Source: CAD feature listing. Evaluate the final solid. Frame: model axes, mm. Face numbers are marked on the shaded views. A direction names the side the tool comes from. Give positions to 0.01 mm unless a question says otherwise; leave off trailing zeros. Order: outer loops, then holes, each group sorted by start corner. A loop starts at its lowest first (then second) coordinate and runs counter-clockwise, first axis right, second up.
1) Access query for the marked faces 4, 5 and 6. Directions: +Z, -Z, +X, -X, +Y, -Y. A direction counts if a zero-diameter tool reaches every point of the face in a straight line with its end or side. Return the directions, or none.
2) First-contact query: P1, Ø13.5, axis at x = 25.15, z = 123.69, coming from the +Y side; P2, Ø2, axis at x = -53.5, z = 72.5, coming from the +Y side; P3, Ø12, axis at y = 124, z = 5, coming from the -X side; P4, Ø8, axis at x = -12.5, y = 18, coming from the -Z side. Flat tips, straight axial feed; report the tip coordinate or a pass-through.
3) Material intervals for line 1 (Y direction, x = 25.5, z = 40); line 2 (Z direction, x = -10, y = 55.5); line 3 (X direction, y = 39.5, z = 27.5), sorted ascending.
4) Section B-B, the plane y = 42. Return loops of the section in (x, z).
5) Draft query along X for the marked faces 1, 2 and 3. Return one class per face: released by +X, released by -X, zero draft, split by the parting line, or undercut.
```python
from build123d import *

# Parameters (mm, degrees)
ESQUISSE1_W             = 170
ESQUISSE1_H             = 170
BOSS_EXTRU_1_DEPTH      = 7
ESQUISSE2_W             = 100
ESQUISSE2_H             = 100
BOSS_EXTRU_2_DEPTH      = 100
COQUE1_START            = 4
COQUE1_OUTLINE_W        = 92
COQUE1_OUTLINE_H        = 92
COQUE1_DEPTH            = 168
COQUE1_START_2          = 138.211102451
COQUE1_2_OUTLINE_R      = 91
COQUE1_2_OUTLINE_W      = 92
COQUE1_2_OUTLINE_H      = 92
COQUE1_2_DEPTH          = 33.788897549
CHANFREIN1_SIZE         = 2
CHANFREIN2_SIZE         = 0.5
ESQUISSE4_R             = 7.5
ENL_V_MAT_EXTRU_1_DEPTH = 70


with BuildPart() as part:
    # Esquisse1 → Boss.-Extru.1 (new body)
    with BuildSketch(Plane(origin=(0, 0, 0), x_dir=(1, 0, 0), z_dir=(0, 1, 0))):
        with Locations((-39.850746269, -58.694029851)):
            Rectangle(ESQUISSE1_W, ESQUISSE1_H)
    extrude(amount=BOSS_EXTRU_1_DEPTH)

    # Esquisse2 → Boss.-Extru.2 (add)
    with BuildSketch(Plane(origin=(0, 7, 0), x_dir=(1, 0, 0), z_dir=(0, 1, 0))):
        with Locations((-39.850746269, -58.694029851)):
            Rectangle(ESQUISSE2_W, ESQUISSE2_H)
    extrude(amount=BOSS_EXTRU_2_DEPTH)

    # Esquisse3 → Révolution1 (revolve)
    with BuildSketch(Plane.XY.offset(60), mode=Mode.PRIVATE) as r_volution1_sk:
        Polygon((55.149253731, 137), (55.149253731, 172), (-39.850746269, 172), (-39.850746269, 107), (35.149253731, 107), align=None)
    revolve(r_volution1_sk.sketch.rotate(Axis((-39.850746269, 172, 60), (0, -1, 0)), 180), axis=Axis((-39.850746269, 172, 60), (0, -1, 0)))

    # Coque1: read off the stored shape, not the designer's step
    # Coque1 outline → Coque1 (cut)
    with BuildSketch(Plane(origin=(0, 0, 0), x_dir=(1, 0, 0), z_dir=(0, 1, 0)).offset(COQUE1_START)):
        with Locations((-39.850746269, -58.694029851)):
            Rectangle(COQUE1_OUTLINE_W, COQUE1_OUTLINE_H)
    extrude(amount=COQUE1_DEPTH, mode=Mode.SUBTRACT)

    # Coque1 2 outline → Coque1 2 (cut)
    with BuildSketch(Plane(origin=(0, 0, 0), x_dir=(1, 0, 0), z_dir=(0, 1, 0)).offset(COQUE1_START_2)):
        with Locations((-39.850746269, -60)):
            Circle(COQUE1_2_OUTLINE_R)
        with Locations((-39.850746269, -58.694029851)):
            Rectangle(COQUE1_2_OUTLINE_W, COQUE1_2_OUTLINE_H, mode=Mode.SUBTRACT)
    extrude(amount=COQUE1_2_DEPTH, mode=Mode.SUBTRACT)

    # Coque1 3 outline → Coque1 3 (revolve, cut)
    with BuildSketch(Plane(origin=(-39.850746269, 0, 60), x_dir=(1, 0, 0), z_dir=(0, 0, 1))):
        Polygon((44.694029851, 138.211102551), (44.694029851, 111), (72.859264966, 111), (91, 138.211102551), align=None)
    revolve(axis=Axis((-39.850746269, 0, 60), (0, 1, 0)), mode=Mode.SUBTRACT)

    # Chanfrein1
    chanfrein1_edges = [part.edges().sort_by_distance(p)[0] for p in [
        (45.149253731, 7, 58.694029851),
        (-89.850746269, 7, 58.694029851),
        (-39.850746269, 7, 108.694029851),
        (10.149253731, 7, 58.694029851),
        (-39.850746269, 7, 8.694029851),
        (-39.850746269, 7, -26.305970149),
        (-124.850746269, 7, 58.694029851),
        (-39.850746269, 7, 143.694029851),
    ]]
    chamfer(chanfrein1_edges, length=CHANFREIN1_SIZE)

    # Chanfrein2
    chanfrein2_edges = [part.edges().sort_by_distance(p)[0] for p in [
        (55.149253731, 172, 60),
        (-130.850746269, 172, 60),
    ]]
    chamfer(chanfrein2_edges, length=CHANFREIN2_SIZE)

    # Esquisse4 → Enlèv. mat.-Extru.1 (cut)
    with BuildSketch(Plane(origin=(0, 7, 0), x_dir=(1, 0, 0), z_dir=(0, 1, 0))):
        with Locations(Location((25.149253731, -123.694029851, 0), (0, 0, 270))):
            Circle(ESQUISSE4_R)
        with Locations(Location((25.149253731, 3.694029851, 0), (0, 0, 270))):
            Circle(ESQUISSE4_R)
        with Locations(Location((-104.850746269, -123.694029851, 0), (0, 0, 270))):
            Circle(ESQUISSE4_R)
        with Locations(Location((-104.850746269, 3.694029851, 0), (0, 0, 270))):
            Circle(ESQUISSE4_R)
    extrude(amount=-ENL_V_MAT_EXTRU_1_DEPTH, mode=Mode.SUBTRACT)


solid = part.part
```
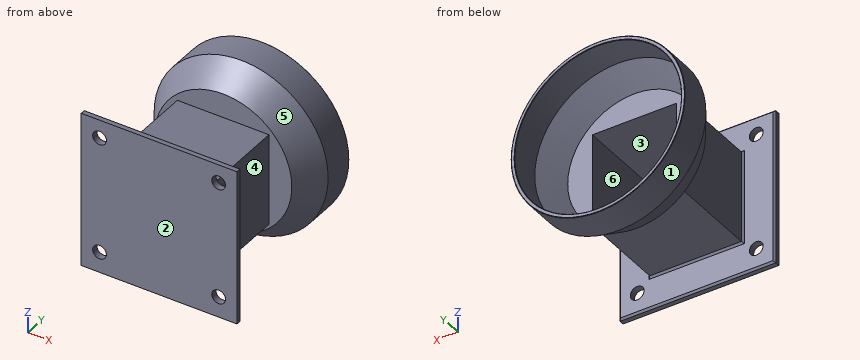
From the geometry:
1. face 4: +Z, -Z, +X
1. face 5: none
1. face 6: +Y
2. P1: stops at y = 172
2. P2: stops at y = 4
2. P3: stops at x = -113.17
2. P4: stops at z = 8.69
3. line 1: y = 0 to 7, 107 to 111
3. line 2: z = 8.69 to 12.69, 104.69 to 108.69
3. line 3: x = -89.85 to -85.85, 6.15 to 10.15
4. outline: (-89.85, 8.69) - (10.15, 8.69) - (10.15, 108.69) - (-89.85, 108.69) - close; hole (-85.85, 12.69) - (6.15, 12.69) - (6.15, 104.69) - (-85.85, 104.69) - close
5. face 1: split by the parting line
5. face 2: zero draft
5. face 3: undercut
